from build123d import *
from OCP.BRepFilletAPI import BRepFilletAPI_MakeChamfer

# Parameters (mm, degrees)
CHAMFER1_SIZE  = 0.1
CHAMFER1_SIZE2 = 0.076325766


with BuildPart() as part:
    # Sketch2 → Revolve1 (revolve)
    with BuildSketch(Plane.XY, mode=Mode.PRIVATE) as revolve1_sk:
        with BuildLine():
            Line((-11, -3.5), (-11, 3.5))
            Line((-11, 3.5), (-8.291561976, 3.5))
            ThreePointArc((-8.291561976, 3.5), (-9, 0), (-8.291561976, -3.5))
            Line((-8.291561976, -3.5), (-11, -3.5))
        make_face()
    revolve(revolve1_sk.sketch.rotate(Axis((0, 0, 0), (0, 1, 0)), 270), axis=Axis((0, 0, 0), (0, 1, 0)))

    # Chamfer1: one chamfer whose edges measure the first distance from different faces: ONE call of the kernel's chamfer builder (chamfer() names one face for all edges)
    chamfer1_edges_1 = [part.edges().sort_by_distance(p)[0] for p in [
        (0, 3.5, 8.291561976),
    ]]
    chamfer1_side_1 = [part.faces().sort_by_distance(p)[0] for p in [
        (0, 0, 9),
    ]]
    chamfer1_edges_2 = [part.edges().sort_by_distance(p)[0] for p in [
        (0, -3.5, 8.291561976),
    ]]
    chamfer1_side_2 = [part.faces().sort_by_distance(p)[0] for p in [
        (0, -3.5, 8.60268896),
    ]]
    chamfer1_edges_3 = [part.edges().sort_by_distance(p)[0] for p in [
        (0, -3.5, 11),
        (0, 3.5, 11),
    ]]
    chamfer1 = BRepFilletAPI_MakeChamfer(part.part.solid().wrapped)
    for e in chamfer1_edges_1:
        chamfer1.Add(CHAMFER1_SIZE, CHAMFER1_SIZE2, e.wrapped, chamfer1_side_1[0].wrapped)  # the first distance lies on this face
    for e in chamfer1_edges_2:
        chamfer1.Add(CHAMFER1_SIZE, CHAMFER1_SIZE2, e.wrapped, chamfer1_side_2[0].wrapped)  # the first distance lies on this face
    for e in chamfer1_edges_3:
        chamfer1.Add(CHAMFER1_SIZE, e.wrapped)
    add(Compound.cast(chamfer1.Shape()), mode=Mode.REPLACE)


solid = part.part
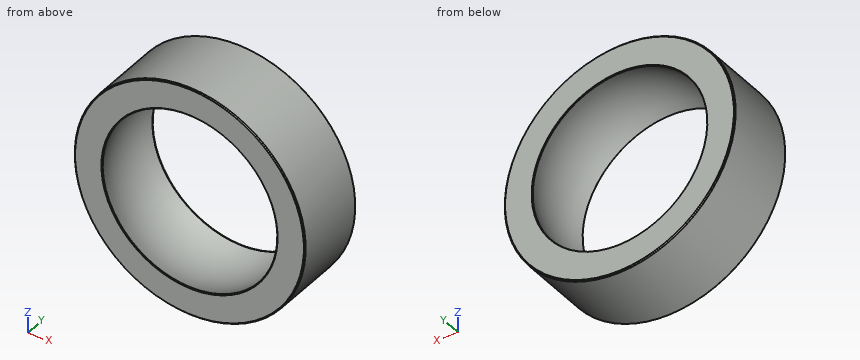
Here's how the part is built. I have some questions about the finished solid (model axes, mm). Coordinates: 2 decimals unless noted, no trailing zeros. Write each loop counter-clockwise with the first axis right and the second up, starting at its lowest first coordinate (ties: lowest second). Pieces come first, ordered by that corner, then holes.
Item 1: I want a section at A-A on y = 2.25. Write out the boundary of the cut face in (x, z).
Item 2: If I drill on line 1 (Z direction, x = 2.5, y = -0.75); line 2 (Z direction, x = -7.5, y = 1); line 3 (Y direction, x = 5, z = -6.75), over which ranges is the centre line in solid material (lowest first)?
Item 3: I want a section at B-B on y = -2.5. Write out the boundary of the cut face in (x, z).
Item 4: Will these pins go through, and if not, where does the flat tip stop? pin 1 (4 mm diameter, centred on y = 2.5, z = 6, fed in from +X); pin 2 (4 mm diameter, centred on x = 2.5, y = 1.5, fed in from +Z); pin 3 (1 mm diameter, centred on x = 3, y = -2, fed in from +Z).
Findings below:
1. outline: circle Ø22 at (0, 0); hole circle Ø17.43 at (0, 0)
2. line 1: z = -10.71 to -8.61, 8.61 to 10.71
2. line 2: z = -8.05 to -4.87, 4.87 to 8.05
2. line 3: y = -3.5 to -3.23, 3.23 to 3.5
3. outline: circle Ø22 at (0, 0); hole circle Ø17.29 at (0, 0)
4. pin 1: stops at x = 10.25
4. pin 2: stops at z = 10.99
4. pin 3: stops at z = 10.71
